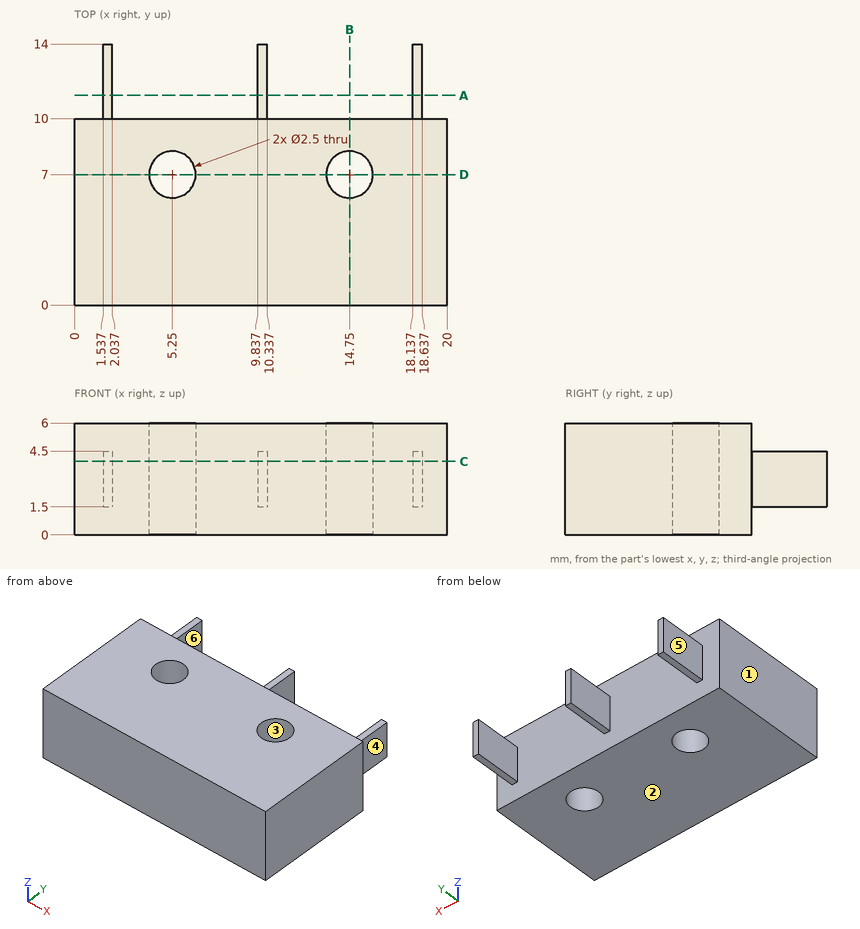
Here's the drawing with two shaded views (mm, measured from the low corner). I have some questions. A direction names the side the tool comes from. Give positions to 0.01 mm unless a question says otherwise; leave off trailing zeros. Order: outer loops, then holes, each group sorted by start corner. A loop starts at its lowest first (then second) coordinate and runs counter-clockwise, first axis right, second up. Notation, with made-up numbers: (34, -13.75) - (84, -13.75) arc R17 cw to (84, 9.25) - close; hole circle Ø7 at (18.25, -3.5). An arc over 180 degrees is marked (long way). Use a Markdown table: item, result. Add a question column.
Q1. I'm going to push flat-ended pins straight in: pin 1 (0.9 mm diameter, centred on y = 12.5, z = 3, fed in from -X); pin 2 (2.5 mm diameter, centred on y = 11.5, z = 2.5, fed in from +X); pin 3 (0.6 mm diameter, centred on x = 1.5, y = 11.5, fed in from +Z); pin 4 (1.5 mm diameter, centred on x = 18, z = 2.5, fed in from -Y). Where does each tip first touch, or does it pass through?
Q2. If we section it at B-B on x = 14.75: Write out the boundary of the cut face in (y, z), plus the area to 3 significant figures.
Q3. If we section it at A-A on y = 11.25: Write out the boundary of the cut face in (x, z).
Q4. Please list where these lines run through material, in increasing order: line 1 along X through (y, z) = (10.25, 2.2); line 2 along Y through (x, z) = (14.75, 1.9); line 3 along Y through (x, z) = (9.25, 4.3).
Q5. If we section it at C-C on z = 3.95: Write out the boundary of the cut face in (x, y).
Q6. On a 3-axis mill with a long thin cutter (end or side, diameter ignored), from which of +Z, -Z, +X, -X, +Y, -Y can I reach the whole of each face in a straight line? I mean the marked faces 4, 5 and 6. Say none if no direction works.
Q7. If we section it at D-D on y = 7: Write out the boundary of the cut face in (x, z).
Q8. If we mould it in two halves opening along X, with no side actions, what happens to the marked faces 1, 2 and 3? For each: released by +X, released by -X, zero draft, split by the parting line, or undercut.
Answers follow:
| question | item | result |
|---|---|---|
| 1 | pin 1 | stops at x = 1.54 |
| 1 | pin 2 | stops at x = 18.64 |
| 1 | pin 3 | stops at z = 4.5 |
| 1 | pin 4 | stops at y = 0 |
| 2 | outline | (0, 0) - (5.75, 0) - (5.75, 6) - (0, 6) - close; (8.25, 0) - (10, 0) - (10, 6) - (8.25, 6) - close |
| 2 | area | 45.0 mm^2 |
| 3 | outline | (1.54, 1.5) - (2.04, 1.5) - (2.04, 4.5) - (1.54, 4.5) - close; (9.84, 1.5) - (10.34, 1.5) - (10.34, 4.5) - (9.84, 4.5) - close; (18.14, 1.5) - (18.64, 1.5) - (18.64, 4.5) - (18.14, 4.5) - close |
| 4 | line 1 | x = 1.54 to 2.04, 9.84 to 10.34, 18.14 to 18.64 |
| 4 | line 2 | y = 0 to 5.75, 8.25 to 10 |
| 4 | line 3 | y = 0 to 10 |
| 5 | outline | (0, 0) - (20, 0) - (20, 10) - (18.64, 10) - (18.64, 14) - (18.14, 14) - (18.14, 10) - (10.34, 10) - (10.34, 14) - (9.84, 14) - (9.84, 10) - (2.04, 10) - (2.04, 14) - (1.54, 14) - (1.54, 10) - (0, 10) - close; hole circle Ø2.5 at (5.25, 7); hole circle Ø2.5 at (14.75, 7) |
| 6 | face 4 | +Z, -Z, +X, +Y |
| 6 | face 5 | +Z, -Z, -X, +Y |
| 6 | face 6 | +Z, -Z, +Y |
| 7 | outline | (0, 0) - (4, 0) - (4, 6) - (0, 6) - close; (6.5, 0) - (13.5, 0) - (13.5, 6) - (6.5, 6) - close; (16, 0) - (20, 0) - (20, 6) - (16, 6) - close |
| 8 | face 1 | released by -X |
| 8 | face 2 | zero draft |
| 8 | face 3 | undercut |
